Read the model definition and answer for the solid it produces. Units are mm, in the model's axes. Face numbers are marked on the shaded views. A direction names the side the tool comes from. Coordinates: 2 decimals unless noted, no trailing zeros. Loops run counter-clockwise (first coordinate to the right, second up) from the corner with the lowest first, then second, coordinate; pieces in that order, holes last.
from build123d import *

# Parameters (mm, degrees)
F0_W     = 273.05
F0_H     = 114.3
F1_DEPTH = 19.05
F2_R     = 38.1
F3_DEPTH = 25.4
F5_DEPTH = 45.72
F7_DEPTH = 25.4


with BuildPart() as f1:
    # F0 (on Front) → F1 (new body)
    with BuildSketch(Plane.XZ):
        with Locations((136.525, 57.15)):
            Rectangle(F0_W, F0_H)
    extrude(amount=F1_DEPTH)

    # F2 (on face) → F3 (cut)
    with BuildSketch(Plane.XZ.offset(19.05)):
        with Locations((47.625, 50.8)):
            Circle(F2_R)
        with Locations((225.425, 50.8)):
            Circle(F2_R)
    extrude(amount=-F3_DEPTH, mode=Mode.SUBTRACT)

    # F4 (on face) → F5 (cut)
    with BuildSketch(Plane.XZ.offset(19.05)):
        with BuildLine():
            Line((177.8, 114.3), (95.25, 114.3))
            Line((95.25, 114.3), (95.25, 49.53))
            ThreePointArc((95.25, 49.53), (98.597769, 41.447769), (106.68, 38.1))
            Line((106.68, 38.1), (166.37, 38.1))
            ThreePointArc((166.37, 38.1), (174.452231, 41.447769), (177.8, 49.53))
            Line((177.8, 49.53), (177.8, 114.3))
        make_face()
    extrude(amount=-F5_DEPTH, mode=Mode.SUBTRACT)

    # F6 (on face) → F7 (cut)
    with BuildSketch(Plane.XZ.offset(19.05)):
        Polygon((166.37, 25.401815), (166.37, 38.1), (140.97, 38.1), (140.97, 25.401815), (59.75961, 25.401815), (47.996878, 12.701815), (225.796878, 12.701815), (196.839669, 25.401815), align=None)
    extrude(amount=-F7_DEPTH, mode=Mode.SUBTRACT)


solid = f1.part
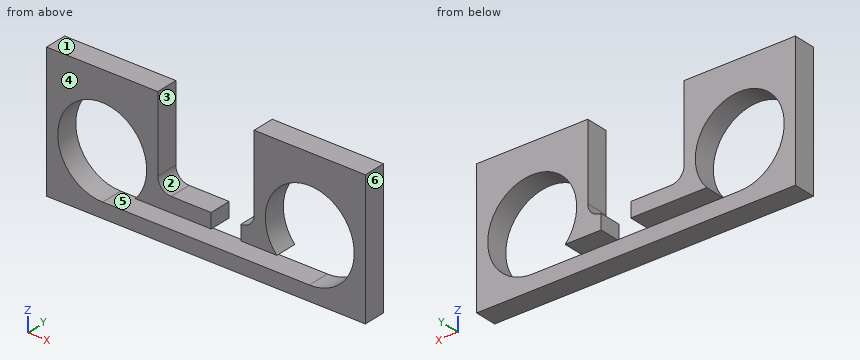
Q1. A cutting plane is placed at C-C (y = -11.5). Give the vertices of the cut face in (x, z) (3 decimals), then the cut area to 3 significant figures.
Findings below:
outline: (0, 0) - (273.05, 0) - (273.05, 114.3) - (177.8, 114.3) - (177.8, 49.53) arc R11.43 cw to (166.37, 38.1) - (166.37, 25.402) - (196.84, 25.402) - (197.146, 25.267) arc R38.1 cw (long way) to (225.053, 12.702) - (47.997, 12.702) arc R38.1 cw (long way) to (76.025, 25.402) - (140.97, 25.402) - (140.97, 38.1) - (106.68, 38.1) arc R11.43 cw to (95.25, 49.53) - (95.25, 114.3) - (0, 114.3) - close
area: 13,800 mm2
Q2. Which of the six approach directions +Z, -Z, +X, -X, +Y, -Y give full straight-line access (tool end or side, diameter ignored) to the marked faces 1 and 2?
Findings below:
face 1: +Z, +X, -X, +Y, -Y
face 2: +Z, +Y, -Y
Q3. Determine the mould class of the marked faces 3, 4, 5 and 6 for opening direction X: +X half, -X half, draft (parallel to the pull), parting line (faces both ways), or undercut.
Findings below:
face 3: undercut
face 4: draft
face 5: undercut
face 6: +X half
Q4. A cutting plane is placed at D-D (z = 72.5). Give the vertices of the cut face in (x, y), then the cut area to 3 significant figures.
Findings below:
outline: (0, -19.05) - (16.31, -19.05) - (16.31, 0) - (0, 0) - close; (78.94, -19.05) - (95.25, -19.05) - (95.25, 0) - (78.94, 0) - close; (177.8, -19.05) - (194.11, -19.05) - (194.11, 0) - (177.8, 0) - close; (256.74, -19.05) - (273.05, -19.05) - (273.05, 0) - (256.74, 0) - close
area: 1,240 mm2
Q5. A flat-ended cylindrical pin translates along its axis: pin 1 Ø6 at (x, y) = (140, -9.5) entering from +Z. Find the tip coordinate at first contact, or state that the pin passes through.
Findings below:
pin 1: stops at z = 38.1
Q6. A cutting plane is placed at B-B (x = 42). Give the vertices of the cut face in (y, z), then the cut area to 3 significant figures.
Findings below:
outline: (-19.05, 0) - (0, 0) - (0, 13.12) - (-19.05, 13.12) - close; (-19.05, 88.48) - (0, 88.48) - (0, 114.3) - (-19.05, 114.3) - close
area: 742 mm2
Q7. Straight lines are drawn through the part: probe 1 along X at (y, z) = (-11, 50.8) (3 decimals); probe 2 along X at (y, z) = (-10.5, 49.5); probe 3 along Z at (x, y) = (90, -14.5). For each, find the intervals that lie inside material, in ascending order.
Findings below:
probe 1: x = 0 to 9.525, 85.725 to 95.25, 177.8 to 187.325, 263.525 to 273.05
probe 2: x = 0 to 9.55, 85.7 to 95.25, 177.8 to 187.35, 263.5 to 273.05
probe 3: z = 0 to 12.7, 25.4 to 114.3
Q8. A cutting plane is placed at A-A (z = 97). Give the vertices of the cut face in (x, y).
Findings below:
outline: (0, -19.05) - (95.25, -19.05) - (95.25, 0) - (0, 0) - close; (177.8, -19.05) - (273.05, -19.05) - (273.05, 0) - (177.8, 0) - close
